Part model, mm, in its own coordinate system. Face numbers are marked on the shaded views. A direction names the side the tool comes from. Round coordinates to 2 decimals unless told otherwise and drop trailing zeros. Loops run counter-clockwise (first coordinate to the right, second up) from the corner with the lowest first, then second, coordinate; pieces in that order, holes last.
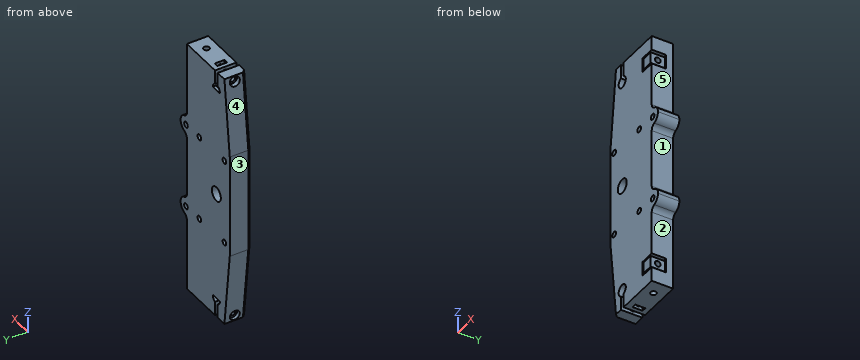
from build123d import *
from build123d.topology import SkipClean

# Parameters (mm, degrees)
SZKIC1_R                    = 2
DODANIE_WYCI_GNI_CIE1_DEPTH = 15
DODANIE_WYCI_GNI_CIE3_START = -2
DODANIE_WYCI_GNI_CIE3_DEPTH = 2
DODANIE_WYCI_GNI_CIE4_DEPTH = 15
WYTNIJ_WYCI_GNI_CIE1_DEPTH  = 15
ZAOKR_GLENIE1_R             = 4
SFAZOWANIE1_SIZE            = 2
WYTNIJ_WYCI_GNI_CIE3_START  = -7
SZKIC8_R                    = 2
WYTNIJ_WYCI_GNI_CIE3_DEPTH  = 107.031560626
WYTNIJ_WYCI_GNI_CIE4_START  = 8
SZKIC9_R                    = 3.5
WYTNIJ_WYCI_GNI_CIE4_DEPTH  = 4
WYTNIJ_WYCI_GNI_CIE5_START  = -6
SZKIC10_R                   = 2
WYTNIJ_WYCI_GNI_CIE5_DEPTH  = 3
SZKIC11_R                   = 2
WYTNIJ_WYCI_GNI_CIE6_DEPTH  = 7
SZKIC12_W                   = 10.2
SZKIC12_H                   = 10.2
SZKIC12_W_2                 = 7.8
SZKIC12_H_2                 = 7.8
WYTNIJ_WYCI_GNI_CIE7_DEPTH  = 10
SZKIC13_R                   = 2
WYTNIJ_WYCI_GNI_CIE8_DEPTH  = 8


with BuildPart() as part:
    # Szkic1 → Dodanie-wyci_gni_cie1 (new body)
    # profile 1 of 2: a face of its own
    with BuildSketch(Plane(origin=(0, 0, 0), x_dir=(1, 0, 0), z_dir=(0, 1, 0))):
        with BuildLine():
            Line((-10.5, 0), (-20.5, 0))
            Line((-20.5, 0), (-20.5, -36.5))
            Line((-20.5, -36.5), (-14.5, -90))
            Line((-14.5, -90), (-7, -90))
            Line((-7, -90), (-7, -80.208099244))
            ThreePointArc((-7, -80.208099244), (-7.736067977, -73.18337521), (-1.5, -76.5))
            ThreePointArc((-1.5, -76.5), (-2.18337521, -78.736067978), (-4, -80.208099244))
            Line((-4, -80.208099244), (-4, -90))
            Line((-4, -90), (27.5, -90))
            Line((27.5, -90), (27.5, 0))
            Line((27.5, 0), (-0.5, 0))
            ThreePointArc((-0.5, 0), (-5.5, -5), (-10.5, 0))
        make_face()
        with Locations(Location((-14.5, -30, 0), (0, 0, 270))):
            Circle(SZKIC1_R, mode=Mode.SUBTRACT)
        with Locations(Location((13.5, -30, 0), (0, 0, 270))):
            Circle(SZKIC1_R, mode=Mode.SUBTRACT)
    # profile 2 of 2: a face of its own
    with BuildSketch(Plane(origin=(0, 0, 0), x_dir=(1, 0, 0), z_dir=(0, 1, 0))):
        with BuildLine():
            Line((-14.5, 90), (-20.5, 36.5))
            Line((-20.5, 36.5), (-20.5, 0))
            Line((-20.5, 0), (-10.5, 0))
            ThreePointArc((-10.5, 0), (-5.5, 5), (-0.5, 0))
            Line((-0.5, 0), (27.5, 0))
            Line((27.5, 0), (27.5, 90))
            Line((27.5, 90), (-3.999999674, 90))
            Line((-3.999999674, 90), (-4, 80.208099244))
            ThreePointArc((-4, 80.208099244), (-2.18337521, 78.736067977), (-1.5, 76.5))
            ThreePointArc((-1.5, 76.5), (-7.736067977, 73.18337521), (-7, 80.208099244))
            Line((-7, 80.208099244), (-6.999999674, 90))
            Line((-6.999999674, 90), (-14.5, 90))
        make_face()
        with Locations(Location((-14.5, 30, 0), (0, 0, 270))):
            Circle(SZKIC1_R, mode=Mode.SUBTRACT)
        with Locations(Location((13.5, 30, 0), (0, 0, 270))):
            Circle(SZKIC1_R, mode=Mode.SUBTRACT)
    extrude(amount=DODANIE_WYCI_GNI_CIE1_DEPTH)

    # Szkic3 → Dodanie-wyci_gni_cie3 (add)
    with BuildSketch(Plane(origin=(0, 15, 0), x_dir=(1, 0, 0), z_dir=(0, 1, 0)).offset(DODANIE_WYCI_GNI_CIE3_START)):
        with BuildLine():
            ThreePointArc((-1.5, -76.5), (-5.5, -72.5), (-9.5, -76.5))
            Line((-9.5, -76.5), (-1.5, -76.5))
        make_face()
        with BuildLine():
            Line((-1.5, 76.5), (-9.5, 76.5))
            ThreePointArc((-9.5, 76.5), (-5.5, 72.5), (-1.5, 76.5))
        make_face()
    extrude(amount=DODANIE_WYCI_GNI_CIE3_DEPTH)

    # Szkic4 → Dodanie-wyci_gni_cie4 (add)
    with BuildSketch(Plane(origin=(0, 15, 0), x_dir=(1, 0, 0), z_dir=(0, 1, 0))):
        with BuildLine():
            ThreePointArc((27.5, -28.267949192), (29.5, -28.267949192), (30.5, -30))
            ThreePointArc((30.5, -30), (29.5, -31.732050808), (27.5, -31.732050808))
            Line((27.5, -31.732050808), (27.5, -35.916079783))
            ThreePointArc((27.5, -35.916079783), (32.372983346, -34.582575695), (34.5, -30))
            ThreePointArc((34.5, -30), (32.372983346, -25.417424305), (27.5, -24.083920217))
            Line((27.5, -24.083920217), (27.5, -28.267949192))
        make_face()
        with BuildLine():
            ThreePointArc((27.5, -31.732050808), (26.5, -30), (27.5, -28.267949192))
            Line((27.5, -28.267949192), (27.5, -24.083920217))
            ThreePointArc((27.5, -24.083920217), (22.5, -30), (27.5, -35.916079783))
            Line((27.5, -35.916079783), (27.5, -31.732050808))
        make_face()
        with BuildLine():
            ThreePointArc((27.5, 35.916079783), (22.5, 30), (27.5, 24.083920217))
            Line((27.5, 24.083920217), (27.5, 28.267949192))
            ThreePointArc((27.5, 28.267949192), (26.5, 30), (27.5, 31.732050808))
            Line((27.5, 31.732050808), (27.5, 35.916079783))
        make_face()
        with BuildLine():
            Line((27.5, 28.267949192), (27.5, 24.083920217))
            ThreePointArc((27.5, 24.083920217), (32.372983346, 25.417424305), (34.5, 30))
            ThreePointArc((34.5, 30), (32.372983346, 34.582575695), (27.5, 35.916079783))
            Line((27.5, 35.916079783), (27.5, 31.732050808))
            ThreePointArc((27.5, 31.732050808), (29.5, 31.732050808), (30.5, 30))
            ThreePointArc((30.5, 30), (29.5, 28.267949192), (27.5, 28.267949192))
        make_face()
    extrude(amount=-DODANIE_WYCI_GNI_CIE4_DEPTH)

    # Szkic5 → Wytnij-wyci_gni_cie1 (cut)
    with SkipClean():  # the faces are left unmerged after this step: merging them gives an invalid solid
        with BuildSketch(Plane(origin=(0, 15, 0), x_dir=(1, 0, 0), z_dir=(0, 1, 0))):
            with BuildLine():
                ThreePointArc((27.5, -28.267949192), (30.5, -30), (27.5, -31.732050808))
                Line((27.5, -31.732050808), (27.5, -28.267949192))
            make_face()
            with BuildLine():
                Line((27.5, -28.267949192), (27.5, -31.732050808))
                ThreePointArc((27.5, -31.732050808), (29.5, -31.732050808), (30.5, -30))
                ThreePointArc((30.5, -30), (29.5, -28.267949192), (27.5, -28.267949192))
            make_face()
            with BuildLine():
                ThreePointArc((27.5, -28.267949192), (26.5, -30), (27.5, -31.732050808))
                Line((27.5, -31.732050808), (27.5, -28.267949192))
            make_face()
            with BuildLine():
                Line((27.5, 31.732050808), (27.5, 28.267949192))
                ThreePointArc((27.5, 28.267949192), (29.5, 28.267949192), (30.5, 30))
                ThreePointArc((30.5, 30), (29.5, 31.732050808), (27.5, 31.732050808))
            make_face()
            with BuildLine():
                ThreePointArc((27.5, 31.732050808), (26.5, 30), (27.5, 28.267949192))
                Line((27.5, 28.267949192), (27.5, 31.732050808))
            make_face()
            with BuildLine():
                ThreePointArc((27.5, 31.732050808), (30.5, 30), (27.5, 28.267949192))
                Line((27.5, 28.267949192), (27.5, 31.732050808))
            make_face()
        extrude(amount=-WYTNIJ_WYCI_GNI_CIE1_DEPTH, mode=Mode.SUBTRACT)

    # Zaokr_glenie1
    zaokr_glenie1_edges = [part.edges().sort_by_distance(p)[0] for p in [
        (27.5, 7.5, -24.083920217),
        (27.5, 7.5, -35.916079783),
        (27.5, 7.5, 35.916079783),
        (27.5, 7.5, 24.083920217),
    ]]
    fillet(zaokr_glenie1_edges, radius=ZAOKR_GLENIE1_R)

    # Sfazowanie1
    sfazowanie1_edges = [part.edges().sort_by_distance(p)[0] for p in [
        (-17.5, 0, 63.25),
        (-20.5, 0, 0),
        (-17.5, 0, -63.25),
    ]]
    chamfer(sfazowanie1_edges, length=SFAZOWANIE1_SIZE)

    # Szkic8 → Wytnij-wyci_gni_cie3 (cut)
    with SkipClean():  # the faces are left unmerged after this step: merging them gives an invalid solid
        with BuildSketch(Plane.ZY.offset(4).offset(WYTNIJ_WYCI_GNI_CIE3_START)):
            with Locations((86, 8)):
                Circle(SZKIC8_R)
        wytnij_wyci_gni_cie3 = extrude(amount=WYTNIJ_WYCI_GNI_CIE3_DEPTH, mode=Mode.SUBTRACT)

    # Szkic9 → Wytnij-wyci_gni_cie4 (cut)
    with SkipClean():  # the faces are left unmerged after this step: merging them gives an invalid solid
        with BuildSketch(Plane.ZY.offset(4).offset(WYTNIJ_WYCI_GNI_CIE4_START)):
            with Locations((86, 8)):
                Circle(SZKIC9_R)
        wytnij_wyci_gni_cie4 = extrude(amount=WYTNIJ_WYCI_GNI_CIE4_DEPTH, mode=Mode.SUBTRACT)

    # Szkic10 → Wytnij-wyci_gni_cie5 (cut)
    # profile 1 of 2: a face of its own
    with SkipClean():  # the faces are left unmerged after this step: merging them gives an invalid solid
        with BuildSketch(Plane.ZY.offset(4).offset(WYTNIJ_WYCI_GNI_CIE5_START)):
            Polygon((89, 6.267949192), (89, 9.732050808), (86, 11.464101615), (83, 9.732050808), (83, 6.267949192), (86, 4.535898385), align=None)
            with Locations((86, 8)):
                Circle(SZKIC10_R, mode=Mode.SUBTRACT)
        # profile 2 of 2: a face of its own
        with BuildSketch(Plane.ZY.offset(4).offset(WYTNIJ_WYCI_GNI_CIE5_START)):
            Polygon((90, 11.464101615), (86, 11.464101615), (89, 9.732050808), (89, 6.267949192), (86, 4.535898385), (90, 4.535898385), align=None)
        wytnij_wyci_gni_cie5 = extrude(amount=WYTNIJ_WYCI_GNI_CIE5_DEPTH, mode=Mode.SUBTRACT)

    # Lustro2: Wytnij-wyci_gni_cie3, Wytnij-wyci_gni_cie4, Wytnij-wyci_gni_cie5 across plane
    with SkipClean():  # the faces are left unmerged after this step: merging them gives an invalid solid
        add(wytnij_wyci_gni_cie3.mirror(Plane.XY), mode=Mode.SUBTRACT)
        add(wytnij_wyci_gni_cie4.mirror(Plane.XY), mode=Mode.SUBTRACT)
        add(wytnij_wyci_gni_cie5.mirror(Plane.XY), mode=Mode.SUBTRACT)

    # Szkic11 → Wytnij-wyci_gni_cie6 (cut)
    with SkipClean():  # the faces are left unmerged after this step: merging them gives an invalid solid
        with BuildSketch(Plane.XY.offset(90)):
            with Locations((17.5, 7.5)):
                Circle(SZKIC11_R)
        wytnij_wyci_gni_cie6 = extrude(amount=-WYTNIJ_WYCI_GNI_CIE6_DEPTH, mode=Mode.SUBTRACT)

    # Lustro3: Wytnij-wyci_gni_cie6 across plane
    with SkipClean():  # the faces are left unmerged after this step: merging them gives an invalid solid
        add(wytnij_wyci_gni_cie6.mirror(Plane.XY), mode=Mode.SUBTRACT)

    # Szkic12 → Wytnij-wyci_gni_cie7 (cut)
    # profile 1 of 2: a face of its own
    with SkipClean():  # the faces are left unmerged after this step: merging them gives an invalid solid
        with BuildSketch(Plane.XZ):
            with Locations((22.4, 74.9)):
                Rectangle(SZKIC12_W, SZKIC12_H)
            with Locations((22.4, 74.9)):
                Rectangle(SZKIC12_W_2, SZKIC12_H_2, mode=Mode.SUBTRACT)
        # profile 2 of 2: a face of its own
        with BuildSketch(Plane.XZ):
            with Locations((22.4, -74.9)):
                Rectangle(SZKIC12_W, SZKIC12_H)
            with Locations((22.4, -74.9)):
                Rectangle(SZKIC12_W_2, SZKIC12_H_2, mode=Mode.SUBTRACT)
        extrude(amount=-WYTNIJ_WYCI_GNI_CIE7_DEPTH, mode=Mode.SUBTRACT)

    # Szkic13 → Wytnij-wyci_gni_cie8 (cut)
    with SkipClean():  # the faces are left unmerged after this step: merging them gives an invalid solid
        with BuildSketch(Plane(origin=(26.3, 0, 0), x_dir=(0, 0, -1), z_dir=(1, 0, 0))):
            with Locations((74.9, 5)):
                Circle(SZKIC13_R)
            with Locations((-74.9, 5)):
                Circle(SZKIC13_R)
        extrude(amount=-WYTNIJ_WYCI_GNI_CIE8_DEPTH, mode=Mode.SUBTRACT)


solid = part.part
1) Wall check: line 1 along Z through (x, y) = (12.5, 7.5); line 2 along Z through (x, y) = (-5.5, 10.75); line 3 along Z through (x, y) = (28.5, 4.5). Give the ranges that are in metal, low to high.
Values:
line 1: z = -90 to -31.73, -28.27 to 28.27, 31.73 to 90
line 2: z = -72.5 to -5, 5 to 72.5
line 3: z = -36.89 to -32, -28 to -23.11, 23.11 to 28, 32 to 36.89
2) Slice it at A-A, the plane x = 13.5. Give the cut face in (y, z), then the cut area to 3 significant figures.
Values:
outline: (0, -90) - (15, -90) - (15, -32) - (0, -32) - close; (0, -28) - (15, -28) - (15, 28) - (0, 28) - close; (0, 32) - (15, 32) - (15, 90) - (0, 90) - close
area: 2,580 mm2
3) Slice it at C-C, the plane z = 74.9. Give the cut face in (x, y), then the cut area to 3 significant figures.
Values:
outline: (-16.19, 2) - (-14.18, 0) - (-9.17, 0) - (-9.17, 13) - (-1.83, 13) - (-1.83, 0) - (17.3, 0) - (17.3, 10) - (18.5, 10) - (18.5, 7) - (26.3, 7) - (26.3, 10) - (27.5, 10) - (27.5, 15) - (-16.19, 15) - close; (18.5, 0) - (26.3, 0) - (26.3, 3) - (18.5, 3) - close
area: 503 mm2
4) Drop flat-ended pins along their axis: pin 1 Ø2 at (x, y) = (-5.5, 14) entering from +Z; pin 2 Ø2 at (y, z) = (6, 9) entering from +X; pin 3 Ø3.5 at (y, z) = (8.5, 86) entering from -X. Give the stop position or say it passes through.
Values:
pin 1: stops at z = 76.5
pin 2: stops at x = 27.5
pin 3: stops at x = -12
5) Slice it at B-B, the plane z = 0. Give the cut face in (x, y).
Values:
outline: (-20.5, 2) - (-18.5, 0) - (-10.5, 0) - (-10.5, 15) - (-20.5, 15) - close; (-0.5, 0) - (27.5, 0) - (27.5, 15) - (-0.5, 15) - close
6) Tool access for the marked faces 1, 2, 3, 4 and 5: list every direction of +Z, -Z, +X, -X, +Y, -Y with a clear straight run to the whole face (end or side of a thin tool).
Values:
face 1: +X, +Y, -Y
face 2: -Z, +X, +Y, -Y
face 3: +Z, -Z, -X, +Y, -Y
face 4: +Z, -X, +Y, -Y
face 5: +Z, +X, +Y, -Y
